from build123d import *

# Parameters (mm, degrees)
SKETCH1_W           = 35.56
SKETCH1_H           = 50.8
BOSS_EXTRUDE1_DEPTH = 20.32
SKETCH2_W           = 49.3776
SKETCH2_H           = 39.2176
CUT_EXTRUDE1_DEPTH  = 34.1376
SKETCH3_R           = 1.27
CUT_EXTRUDE2_DEPTH  = 2.4224
CUT_EXTRUDE3_DEPTH  = 2.4224
SKETCH7_R           = 11.1506
SKETCH7_R_2         = 1.5875
CUT_EXTRUDE4_DEPTH  = 2.4224


with BuildPart() as part:
    # Sketch1 → Boss-Extrude1 (new body, symmetric)
    with BuildSketch(Plane(origin=(0, 0, 0), x_dir=(1, 0, 0), z_dir=(0, 1, 0))):
        Rectangle(SKETCH1_W, SKETCH1_H)
    extrude(amount=BOSS_EXTRUDE1_DEPTH, both=True)

    # Sketch2 → Cut-Extrude1 (cut)
    with BuildSketch(Plane(origin=(17.78, 0, 0), x_dir=(0, 0, -1), z_dir=(1, 0, 0))):
        with Locations((0.7112, 0.7112)):
            Rectangle(SKETCH2_W, SKETCH2_H)
    extrude(amount=-CUT_EXTRUDE1_DEPTH, mode=Mode.SUBTRACT)

    # Sketch3 → Cut-Extrude2 (cut, through all)
    with BuildSketch(Plane(origin=(0, -18.8976, 0), x_dir=(1, 0, 0), z_dir=(0, 1, 0))):
        with Locations((-5.08, -8.89)):
            Circle(SKETCH3_R)
        with Locations((10.16, -8.89)):
            Circle(SKETCH3_R)
        with Locations((-5.08, 12.7)):
            Circle(SKETCH3_R)
    extrude(amount=-CUT_EXTRUDE2_DEPTH, mode=Mode.SUBTRACT)

    # Sketch6 → Cut-Extrude3 (cut, through all)
    with BuildSketch(Plane(origin=(0, 0, 23.9776), x_dir=(-1, 0, 0), z_dir=(0, 0, -1))):
        with BuildLine():
            Line((-17.78, -13.335), (-17.78, 20.32))
            Line((-17.78, 20.32), (10.16, 20.32))
            Line((10.16, 20.32), (10.16, -5.715))
            ThreePointArc((10.16, -5.715), (7.928153673, -11.103153673), (2.54, -13.335))
            Line((2.54, -13.335), (-17.78, -13.335))
        make_face()
    extrude(amount=-CUT_EXTRUDE3_DEPTH, mode=Mode.SUBTRACT)

    # Sketch7 → Cut-Extrude4 (cut, through all)
    with BuildSketch(Plane(origin=(-16.3576, 0, 0), x_dir=(0, 0, -1), z_dir=(1, 0, 0))):
        with Locations((2.3114, -0.9906)):
            Circle(SKETCH7_R)
        with Locations((-12.9286, 14.2494)):
            Circle(SKETCH7_R_2)
        with Locations((17.5514, 14.2494)):
            Circle(SKETCH7_R_2)
        with Locations((17.5514, -16.2306)):
            Circle(SKETCH7_R_2)
        with Locations((-12.9286, -16.2306)):
            Circle(SKETCH7_R_2)
    extrude(amount=-CUT_EXTRUDE4_DEPTH, mode=Mode.SUBTRACT)


solid = part.part
Can you work these out from the model? Positions are in its coordinate system, mm. A direction names the side the tool comes from. Coordinates: 2 decimals unless noted, no trailing zeros. Loops run counter-clockwise (first coordinate to the right, second up) from the corner with the lowest first, then second, coordinate; pieces in that order, holes last. Notation, with made-up numbers: M 51.5,21 L 99.5,21 A25 ccw 99.5,48 Z; hole C 51.25,-36.75 d3. An arc over 180 degrees is marked long. Answer as CSV lines item,"result". Start each with the question number.
1. Suppose I cut it at A-A, the plane x = 10.16. List the corners of the cut face in (y, z) for me (3 decimals).
2. Thinking about a two-plate mould opening in Y: for faces 1 (the face through (-17, 20.32, 4)), 2 (the face through (-10.16, 7, 25)), 3 (the face through (-17.06, 12.84, -18.28)), which applies, +Y half, -Y half, draft (parallel to the pull), parting line (faces both ways), or undercut?
3. Suppose I cut it at B-B, the plane y = -10.5. List the corners of the cut face in (x, z) for me, plus the area to 3 significant figures.
4. Suppose I cut it at C-C, the plane z = -12.7. List the corners of the cut face in (x, y) for me.
5. If I drill on probe 1 along X at (y, z) = (-19.8, 8.89); probe 2 along Y at (x, z) = (-7.5, 19.5); probe 3 along X at (y, z) = (11, -16), over which ranges is the centre line in solid material (lowest first)? Write a range as [from, to].
6. For faces 4 (the face through (-11, -7, 23.978)), 5 (the face through (7, -13.335, 25)), 6 (the face through (-3.87, -19.6, 8.51)), which set-ups out of +Z, -Z, +X, -X, +Y, -Y let a thin tool reach every point of the face, with its end or its side?
7. Suppose I cut it at D-D, the plane x = -5.08. List the corners of the cut face in (y, z) for me, plus the area to 3 significant figures.
8. For pin 1 Ø1.9 at (y, z) = (-16.23, 12.93) entering from -X; pin 2 Ø8 at (x, y) = (-6.5, -6.5) entering from -Z; pin 3 Ø1.6 at (x, z) = (6, 24.5) entering from +Y (3 decimals); pin 4 Ø0.7 at (y, z) = (5, 24.5) entering from +X, each with a flat end and sliding along its axis, tell me the tip position at first contact or that it passes through.
Output:
1,outline,"M -20.32,-25.4 L -18.898,-25.4 L -18.898,7.62 L -20.32,7.62 Z; M -20.32,10.16 L -18.898,10.16 L -18.898,23.978 L -13.335,23.978 L -13.335,25.4 L -20.32,25.4 Z"
2,face 1,"+Y half"
2,face 2,"draft"
2,face 3,"undercut"
3,outline,"M -17.78,-25.4 L -16.36,-25.4 L -16.36,-8.13 L -17.78,-8.13 Z; M -17.78,3.51 L -16.36,3.51 L -16.36,23.98 L -8.47,23.98 L -8.47,25.4 L -17.78,25.4 Z"
3,area,"66.9 mm^2"
4,outline,"M -17.78,-20.32 L -6.35,-20.32 L -6.35,-18.9 L -16.36,-18.9 L -16.36,-5.04 L -17.78,-5.04 Z; M -17.78,3.06 L -16.36,3.06 L -16.36,20.32 L -17.78,20.32 Z; M -3.81,-20.32 L 17.78,-20.32 L 17.78,-18.9 L -3.81,-18.9 Z"
5,probe 1,"x = [-17.78, -6.35], [-3.81, 8.89], [11.43, 17.78]"
5,probe 2,"y = [-20.32, -18.9]"
5,probe 3,"x = [-17.78, -16.36]"
6,face 4,"-Z, +X, +Y"
6,face 5,"+Z, -Z, +X, +Y"
6,face 6,"+Y, -Y"
7,outline,"M -20.32,-25.4 L -18.9,-25.4 L -18.9,-13.97 L -20.32,-13.97 Z; M -20.32,-11.43 L -18.9,-11.43 L -18.9,7.62 L -20.32,7.62 Z; M -20.32,10.16 L -18.9,10.16 L -18.9,23.98 L -12.9,23.98 L -12.9,25.4 L -20.32,25.4 Z"
7,area,"73.6 mm^2"
8,pin 1,"passes through"
8,pin 2,"stops at z = 23.98"
8,pin 3,"stops at y = -13.335"
8,pin 4,"stops at x = -10.16"
